```python
from build123d import *

# Parameters (mm, degrees)
F0_W     = 38.3040010929
F0_H     = 38.1780005991
F1_DEPTH = 38.1
F2_W     = 10.8359996229
F2_H     = 6.5519977361
F2_W_2   = 14.112001285
F2_H_2   = 16.5060013533
F3_DEPTH = 38.1
F5_DEPTH = 38.1
F6_DEPTH = 25.4
F7_DEPTH = 25.4


with BuildPart() as f1:
    # F0 (on Right) → F1 (new body)
    with BuildSketch(Plane.YZ):
        with Locations((19.1520005465, 19.0890002996)):
            Rectangle(F0_W, F0_H)
    extrude(amount=-F1_DEPTH)

    # F2 (on Right) → F3 (cut)
    with BuildSketch(Plane.YZ):
        with Locations((19.0259991214, 26.8379999325)):
            Rectangle(F2_W, F2_H)
        with Locations((18.9000004902, 8.2530006766)):
            Rectangle(F2_W_2, F2_H_2)
    extrude(amount=-F3_DEPTH, mode=Mode.SUBTRACT)

    # F4 (on face) → F5 (cut)
    with BuildSketch(Plane.XZ):
        Polygon((-17.78, 6.426000502), (-8.89, 38.1780005991), (-29.21, 38.1780005991), align=None)
        Polygon((-38.1, 0), (-26.67, 0), (-38.1, 38.1780005991), align=None)
        Polygon((-8.89, 0), (0, 0), (0, 38.1780005991), align=None)
    extrude(amount=-F5_DEPTH, mode=Mode.SUBTRACT)

    # F6 (cut): faces of the model
    f6_faces = [f1.faces().sort_by_distance(p)[0] for p in [
        (-18.6266666667, 38.1, 27.5940005668),
        (-34.29, 38.1, 12.7260001997),
        (-2.9633333333, 38.1, 12.7260001997),
    ]]
    extrude(f6_faces, amount=-F6_DEPTH, mode=Mode.SUBTRACT)

    # F7 (cut): faces of the model
    f7_faces = [f1.faces().sort_by_distance(p)[0] for p in [
        (-4.445, 19.1520005465, 38.1780005991),
        (-33.655, 19.1520005465, 38.1780005991),
    ]]
    extrude(f7_faces, amount=F7_DEPTH, mode=Mode.SUBTRACT)


solid = f1.part
```
Build history of the part. All positions in model axes, mm. A direction names the side the tool comes from. Round coordinates to 2 decimals unless told otherwise and drop trailing zeros. Loops run counter-clockwise (first coordinate to the right, second up) from the corner with the lowest first, then second, coordinate; pieces in that order, holes last.
Item 1: Two-plate mould, pull along X, no slides. Class faces 1 (the face through (-29, 19, 23.562)), 2 (the face through (-13.397, 18.884, 22.08)), 3 (the face through (-4.38, 18.88, 19.36)): released by +X, released by -X, zero draft, split by the parting line, or undercut.
Item 2: Saw through at A-A (z = 36.5). List the corners of the cut face in (x, y).
Item 3: Saw through at D-D (z = 29.5). List the corners of the cut face in (x, y).
Item 4: Saw through at C-C (x = -30). List the corners of the cut face in (y, z).
Item 5: Drill centre lines: line 1 along Y through (x, z) = (-11.5, 26.5); line 2 along Y through (x, z) = (-29, 14); line 3 along Z through (x, y) = (-34, 18). Where is each one in solid material? Low to high.
Item 6: Pin check, flat tips, straight feed: P1, Ø3, axis at x = -26.5, z = 33.5, coming from the -Y side; P2, Ø5, axis at x = -28.5, y = 21, coming from the -Z side; P3, Ø1, axis at y = 25.5, z = 29, coming from the -X side; P4, Ø8, axis at y = 26, z = 17.5, coming from the -X side. Stop position of each tip, or through.
Item 7: Saw through at B-B (y = 19.5). List the corners of the cut face in (x, z).
Item 8: Which spindle directions (+Z, -Z, +X, -X, +Y, -Y) get a long thin tool onto all of the face, cutting with end or side? Do faces 4 (the face through (-30, 13.608, 27)), 5 (the face through (-23.575, 18.884, 22.524)), 6 (the face through (-18, 25.956, 6)). Say none if no direction does.
Worked answers:
1. face 1: zero draft
1. face 2: undercut
1. face 3: released by +X
2. outline: (-37.6, 0) - (-28.61, 0) - (-28.61, 38.3) - (-37.6, 38.3) - close; (-9.36, 0) - (-0.39, 0) - (-0.39, 38.3) - (-9.36, 38.3) - close
3. outline: (-35.5, 0) - (-26.09, 0) - (-26.09, 13.61) - (-35.5, 13.61) - close; (-35.5, 24.44) - (-26.09, 24.44) - (-26.09, 38.3) - (-35.5, 38.3) - close; (-11.32, 0) - (-2.02, 0) - (-2.02, 13.61) - (-11.32, 13.61) - close; (-11.32, 24.44) - (-2.02, 24.44) - (-2.02, 38.3) - (-11.32, 38.3) - close
4. outline: (0, 11.12) - (11.84, 11.12) - (11.84, 16.51) - (25.96, 16.51) - (25.96, 11.12) - (38.3, 11.12) - (38.3, 38.18) - (0, 38.18) - close; hole (13.61, 23.56) - (24.44, 23.56) - (24.44, 30.11) - (13.61, 30.11) - close
5. line 1: y = 0 to 13.61, 24.44 to 38.3
5. line 2: y = 0 to 11.84, 25.96 to 38.3
5. line 3: z = 30.11 to 38.18
6. P1: stops at y = 0
6. P2: stops at z = 16.51
6. P3: stops at x = -35.5
6. P4: stops at x = -33.11
7. outline: (-38.1, 38.18) - (-35.69, 30.11) - (-26.31, 30.11) - (-29.21, 38.18) - close; (-33.72, 23.56) - (-31.61, 16.51) - (-21.41, 16.51) - (-23.95, 23.56) - close; (-14.96, 16.51) - (-5.05, 16.51) - (-3.4, 23.56) - (-12.98, 23.56) - close; (-11.15, 30.11) - (-1.88, 30.11) - (0, 38.18) - (-8.89, 38.18) - close
8. face 4: +X, -X
8. face 5: +Z, +Y, -Y
8. face 6: -Z, +X, -X
